```python
from build123d import *

# Parameters (mm, degrees)
SKETCH1_W                 = 22
SKETCH1_H                 = 4
SKETCH1_R                 = 3
SKETCH1_R_2               = 1.5
BOSS_EXTRUDE1_DEPTH       = 210
SKETCH2_R                 = 1.5
CUT_EXTRUDE2_DEPTH        = 30
LPATTERN1_COUNT           = 3
LPATTERN1_PITCH           = 60
SKETCH5_R                 = 4.5
SKETCH5_R_2               = 1.5
BOSS_EXTRUDE2_DEPTH       = 14
LPATTERN2_COUNT           = 3
LPATTERN2_PITCH           = 60
MIRROR3_COPY_1_SKETCH_R   = 1.5
MIRROR3_COPY_1_DEPTH      = 30
MIRROR3_COPY_2_SKETCH_R   = 1.5
MIRROR3_COPY_2_DEPTH      = 30
MIRROR3_COPY_3_SKETCH_R   = 4.5
MIRROR3_COPY_3_SKETCH_R_2 = 1.5
MIRROR3_COPY_3_DEPTH      = 14
MIRROR3_COPY_4_SKETCH_R   = 4.5
MIRROR3_COPY_4_SKETCH_R_2 = 1.5
MIRROR3_COPY_4_DEPTH      = 14
SKETCH6_R                 = 15
SKETCH6_R_2               = 11
BOSS_EXTRUDE3_DEPTH       = 12
SKETCH9_R                 = 11
CUT_EXTRUDE4_DEPTH        = 40.5
LPATTERN4_COUNT           = 3
LPATTERN4_PITCH           = 75
LPATTERN5_COUNT           = 3
LPATTERN5_PITCH           = 75
BOSS_EXTRUDE4_START       = 6
BOSS_EXTRUDE4_DEPTH       = 6
BOSS_EXTRUDE5_DEPTH       = 3
SKETCH20_W                = 171.257053273
SKETCH20_H                = 66.541862684
CUT_EXTRUDE7_DEPTH        = 6


with BuildPart() as part:
    # Sketch1 → Boss-Extrude1 (new body)
    # profile 1 of 3: a face of its own
    with BuildSketch(Plane.XY):
        with Locations((11, -11.489354466)):
            Rectangle(SKETCH1_W, SKETCH1_H)
    # profile 2 of 3: a face of its own
    with BuildSketch(Plane.XY):
        with BuildLine():
            Line((24.555722734, -8.641839682), (22, -9.489354466))
            Line((22, -9.489354466), (22, -13.489354466))
            Line((22, -13.489354466), (24.555722734, -14.336869249))
            ThreePointArc((24.555722734, -14.336869249), (22.5, -11.489354466), (24.555722734, -8.641839682))
        make_face()
    # profile 3 of 3: a face of its own
    with BuildSketch(Plane.XY):
        with Locations((25.5, -11.489354466)):
            Circle(SKETCH1_R)
        with Locations((25.5, -11.489354466)):
            Circle(SKETCH1_R_2, mode=Mode.SUBTRACT)
    boss_extrude1 = extrude(amount=-BOSS_EXTRUDE1_DEPTH)

    # Sketch2 → Cut-Extrude2 (cut)
    with BuildSketch(Plane.XY.offset(-30)):
        Polygon((22, -6.148469854), (22, -9.489354466), (22, -13.489354466), (22, -16.198394767), (29.348135307, -16.198394767), (29.348135307, -6.148469854), align=None)
        with Locations((25.5, -11.489354466)):
            Circle(SKETCH2_R, mode=Mode.SUBTRACT)
    cut_extrude2 = extrude(amount=-CUT_EXTRUDE2_DEPTH, mode=Mode.SUBTRACT)

    # LPattern1: Cut-Extrude2 ×3
    with Locations(*[(0, 0, -i * LPATTERN1_PITCH) for i in range(1, LPATTERN1_COUNT)]):
        add(cut_extrude2, mode=Mode.SUBTRACT)

    # Sketch5 → Boss-Extrude2 (add)
    # profile 1 of 2: a face of its own
    with BuildSketch(Plane.XY.offset(-38)):
        with BuildLine():
            ThreePointArc((24.1, -6.689354466), (18.020545578, -7.744658151), (16.602885683, -1.739354466))
            Line((16.602885683, -1.739354466), (12.128421097, -9.489354466))
            Line((12.128421097, -9.489354466), (22, -9.489354466))
            Line((22, -9.489354466), (24.1, -6.689354466))
        make_face()
    # profile 2 of 2: a face of its own
    with BuildSketch(Plane.XY.offset(-38)):
        with Locations((20.5, -3.989354466)):
            Circle(SKETCH5_R)
        with Locations((20.5, -3.989354466)):
            Circle(SKETCH5_R_2, mode=Mode.SUBTRACT)
    boss_extrude2 = extrude(amount=-BOSS_EXTRUDE2_DEPTH)

    # LPattern2: Boss-Extrude2 ×3
    with Locations(*[(0, 0, -i * LPATTERN2_PITCH) for i in range(1, LPATTERN2_COUNT)]):
        add(boss_extrude2)

    # Mirror3: Boss-Extrude1, Cut-Extrude2, Boss-Extrude2 across plane
    add(boss_extrude1.mirror(Plane(origin=(0, 0, -210), x_dir=(0, 0, 1), z_dir=(-1, 0, 0))))
    add(cut_extrude2.mirror(Plane(origin=(0, 0, -210), x_dir=(0, 0, 1), z_dir=(-1, 0, 0))), mode=Mode.SUBTRACT)
    add(boss_extrude2.mirror(Plane(origin=(0, 0, -210), x_dir=(0, 0, 1), z_dir=(-1, 0, 0))))

    # Mirror3 copy 1 sketch → Mirror3 copy 1 (cut)
    with BuildSketch(Plane(origin=(0, 0, -90), x_dir=(-1, 0, 0), z_dir=(0, 0, 1))):
        Polygon((22, 6.148469854), (22, 9.489354466), (22, 13.489354466), (22, 16.198394767), (29.348135307, 16.198394767), (29.348135307, 6.148469854), align=None)
        with Locations((25.5, 11.489354466)):
            Circle(MIRROR3_COPY_1_SKETCH_R, mode=Mode.SUBTRACT)
    extrude(amount=-MIRROR3_COPY_1_DEPTH, mode=Mode.SUBTRACT)

    # Mirror3 copy 2 sketch → Mirror3 copy 2 (cut)
    with BuildSketch(Plane(origin=(0, 0, -150), x_dir=(-1, 0, 0), z_dir=(0, 0, 1))):
        Polygon((22, 6.148469854), (22, 9.489354466), (22, 13.489354466), (22, 16.198394767), (29.348135307, 16.198394767), (29.348135307, 6.148469854), align=None)
        with Locations((25.5, 11.489354466)):
            Circle(MIRROR3_COPY_2_SKETCH_R, mode=Mode.SUBTRACT)
    extrude(amount=-MIRROR3_COPY_2_DEPTH, mode=Mode.SUBTRACT)

    # Mirror3 copy 3 sketch → Mirror3 copy 3 (add)
    # profile 1 of 2: a face of its own
    with BuildSketch(Plane(origin=(0, 0, -98), x_dir=(-1, 0, 0), z_dir=(0, 0, 1))):
        with BuildLine():
            ThreePointArc((24.1, 6.689354466), (18.020545578, 7.744658151), (16.602885683, 1.739354466))
            Line((16.602885683, 1.739354466), (12.128421097, 9.489354466))
            Line((12.128421097, 9.489354466), (22, 9.489354466))
            Line((22, 9.489354466), (24.1, 6.689354466))
        make_face()
    # profile 2 of 2: a face of its own
    with BuildSketch(Plane(origin=(0, 0, -98), x_dir=(-1, 0, 0), z_dir=(0, 0, 1))):
        with Locations((20.5, 3.989354466)):
            Circle(MIRROR3_COPY_3_SKETCH_R)
        with Locations((20.5, 3.989354466)):
            Circle(MIRROR3_COPY_3_SKETCH_R_2, mode=Mode.SUBTRACT)
    extrude(amount=-MIRROR3_COPY_3_DEPTH)

    # Mirror3 copy 4 sketch → Mirror3 copy 4 (add)
    # profile 1 of 2: a face of its own
    with BuildSketch(Plane(origin=(0, 0, -158), x_dir=(-1, 0, 0), z_dir=(0, 0, 1))):
        with BuildLine():
            ThreePointArc((24.1, 6.689354466), (18.020545578, 7.744658151), (16.602885683, 1.739354466))
            Line((16.602885683, 1.739354466), (12.128421097, 9.489354466))
            Line((12.128421097, 9.489354466), (22, 9.489354466))
            Line((22, 9.489354466), (24.1, 6.689354466))
        make_face()
    # profile 2 of 2: a face of its own
    with BuildSketch(Plane(origin=(0, 0, -158), x_dir=(-1, 0, 0), z_dir=(0, 0, 1))):
        with Locations((20.5, 3.989354466)):
            Circle(MIRROR3_COPY_4_SKETCH_R)
        with Locations((20.5, 3.989354466)):
            Circle(MIRROR3_COPY_4_SKETCH_R_2, mode=Mode.SUBTRACT)
    extrude(amount=-MIRROR3_COPY_4_DEPTH)

    # Sketch6 → Boss-Extrude3 (add)
    with BuildSketch(Plane(origin=(0, -9.489354466, 0), x_dir=(1, 0, 0), z_dir=(0, 1, 0))):
        with Locations(Location((0, 181.5, 0), (0, 0, 90))):
            Circle(SKETCH6_R)
        with Locations(Location((0, 181.5, 0), (0, 0, 270))):
            Circle(SKETCH6_R_2, mode=Mode.SUBTRACT)
    boss_extrude3 = extrude(amount=BOSS_EXTRUDE3_DEPTH)

    # Sketch9 → Cut-Extrude4 (cut, symmetric)
    with BuildSketch(Plane(origin=(0, -9.489354466, 0), x_dir=(1, 0, 0), z_dir=(0, 1, 0))):
        with Locations(Location((0, 181.5, 0), (0, 0, 90))):
            Circle(SKETCH9_R)
    cut_extrude4 = extrude(amount=CUT_EXTRUDE4_DEPTH, both=True, mode=Mode.SUBTRACT)

    # LPattern4: Boss-Extrude3 ×3
    with Locations(*[(0, 0, i * LPATTERN4_PITCH) for i in range(1, LPATTERN4_COUNT)]):
        add(boss_extrude3)

    # LPattern5: Cut-Extrude4 ×3
    with Locations(*[(0, 0, i * LPATTERN5_PITCH) for i in range(1, LPATTERN5_COUNT)]):
        add(cut_extrude4, mode=Mode.SUBTRACT)

    # Sketch15 → Boss-Extrude4 (add)
    with BuildSketch(Plane.XY.offset(BOSS_EXTRUDE4_START)):
        with BuildLine():
            Line((-22, -9.489354466), (22, -9.489354466))
            Line((22, -9.489354466), (24.555722734, -8.641839682))
            ThreePointArc((24.555722734, -8.641839682), (28.5, -11.489354466), (24.555722734, -14.336869249))
            Line((24.555722734, -14.336869249), (22, -13.489354466))
            Line((22, -13.489354466), (-22, -13.489354466))
            Line((-22, -13.489354466), (-24.555722734, -14.336869249))
            ThreePointArc((-24.555722734, -14.336869249), (-28.5, -11.489354466), (-24.555722734, -8.641839682))
            Line((-24.555722734, -8.641839682), (-22, -9.489354466))
        make_face()
    boss_extrude4 = extrude(amount=-BOSS_EXTRUDE4_DEPTH)

    # Sketch16 → Boss-Extrude5 (add)
    with BuildSketch(Plane.XY.offset(6)):
        Polygon((-22, -13.489354466), (-22, -14.489354466), (-17, -23.489354466), (17, -23.489354466), (22, -14.489354466), (22, -13.489354466), align=None)
    boss_extrude5 = extrude(amount=-BOSS_EXTRUDE5_DEPTH)

    # Mirror6: Boss-Extrude4, Boss-Extrude5 across plane
    add(boss_extrude4.mirror(Plane(origin=(0, 0, -105), x_dir=(1, 0, 0), z_dir=(0, 0, -1))))
    add(boss_extrude5.mirror(Plane(origin=(0, 0, -105), x_dir=(1, 0, 0), z_dir=(0, 0, -1))))

    # Sketch20 → Cut-Extrude7 (cut)
    with BuildSketch(Plane.XY.offset(6)):
        with Locations((-24.250521665, -15.687669002)):
            Rectangle(SKETCH20_W, SKETCH20_H)
    extrude(amount=-CUT_EXTRUDE7_DEPTH, mode=Mode.SUBTRACT)


solid = part.part
```
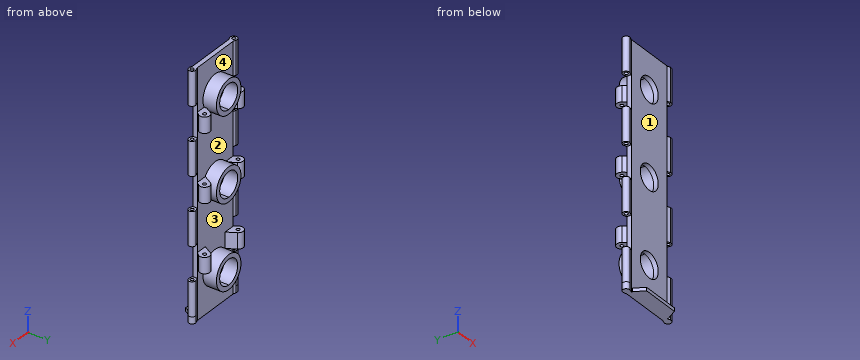
The listing builds one solid part. Answer for the finished solid, in the listing's coordinates (mm). Face numbers are marked on the shaded views. A direction names the side the tool comes from. Coordinates: 2 decimals unless noted, no trailing zeros. Loops run counter-clockwise (first coordinate to the right, second up) from the corner with the lowest first, then second, coordinate; pieces in that order, holes last. Notation, with made-up numbers: (-8.5, 25) -> (7.5, 25) arc R27 cw to (7.5, 48) -> close; hole circle Ø11 at (73.5, -4.5). An arc over 180 degrees is marked (long way). Use one line per item in the form item = value. Start each with the question number.
Item 1: A tool of negligible diameter and unlimited length cuts with its end or side. For the marked faces 1 and 2, from which of +Z, -Z, +X, -X, +Y, -Y can it reach the whole face along a straight path? Write none if from no direction.
Item 2: The mould has two halves that part along X. Classify the marked faces 3 and 4: released by +X, released by -X, zero draft, split by the parting line, or undercut.
Item 3: Consider L1, parallel to Z at x = 23, y = -12.5; L2, parallel to Y at x = -20.5, z = -41.25; L3, parallel to X at y = -10.45, z = -106.5. Determine where each line is inside the solid, lowest interval first. Write a range as [from, to].
Item 4: Flat-ended cylindrical pins translate along their axes: pin 1 Ø4.5 at (y, z) = (-11.5, -164.5) entering from +X; pin 2 Ø8 at (x, y) = (17, -5) entering from +Z; pin 3 Ø3.5 at (x, y) = (-20.5, -3.99) entering from +Z; pin 4 Ø20 at (x, z) = (0, -106.5) entering from -Y (1 decimal). Find the tip coordinate at first contact, or state that the pin passes through.
Item 5: The part is cut by section B-B on z = -132. Determine the outline of the cut face in (x, y).
Item 6: The part is cut by section A-A on z = -106.5. Determine the outline of the cut face in (x, y).
Answer key:
q1.face_1 = +Z, -Y
q1.face_2 = +Y
q2.face_3 = undercut
q2.face_4 = undercut
q3.L1 = [-216, -180], [-150, -120], [-90, -60], [-30, 0]
q3.L2 = [-13.49, -5.49], [-2.49, 0.51]
q3.L3 = [-22, -11], [11, 22]
q4.pin_1 = 22.18
q4.pin_2 = -24.02
q4.pin_3 = -38
q4.pin_4 = through
q5.outline = (-24.56, -14.34) -> (-22, -13.49) -> (22, -13.49) -> (24.56, -14.34) arc R3 ccw (long way) to (24.56, -8.64) -> (22, -9.49) -> (-22, -9.49) -> (-24.56, -8.64) arc R3 ccw (long way) to start; hole circle Ø3 at (-25.5, -11.49); hole circle Ø3 at (25.5, -11.49)
q6.outline = (-24.1, -6.69) -> (-22, -9.49) -> (-22, -13.49) -> (-11, -13.49) -> (-11, 2.51) -> (-15, 2.51) -> (-15, -4.52) -> (-16.6, -1.74) arc R4.5 ccw (long way) to start; (11, -13.49) -> (22, -13.49) -> (22, -9.49) -> (24.1, -6.69) arc R4.5 ccw (long way) to (16.6, -1.74) -> (15, -4.52) -> (15, 2.51) -> (11, 2.51) -> close; hole circle Ø3 at (-20.5, -3.99); hole circle Ø3 at (20.5, -3.99)
